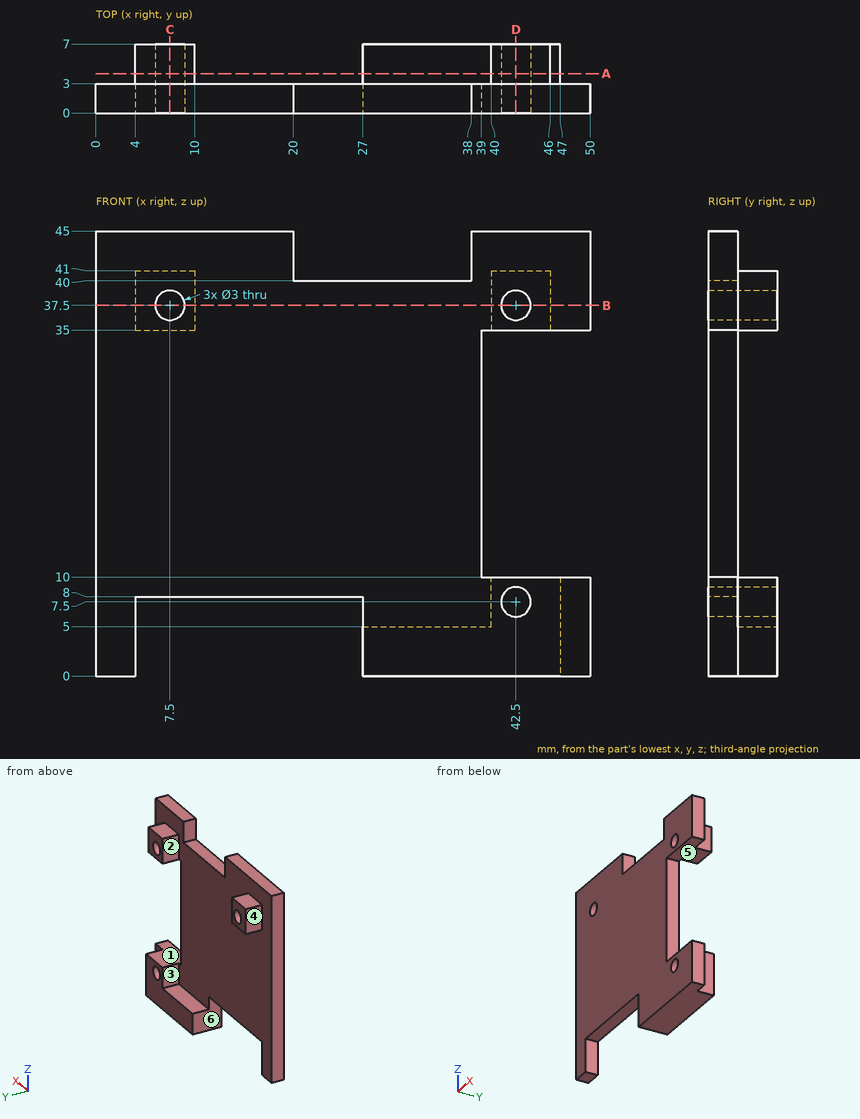
Part print with two shaded views. Sizes in mm from the minimum x, y, z corner. A direction names the side the tool comes from. Give positions to 0.01 mm unless a question says otherwise; leave off trailing zeros. Order: outer loops, then holes, each group sorted by start corner. A loop starts at its lowest first (then second) coordinate and runs counter-clockwise, first axis right, second up. Notation, with made-up numbers: M -40,-28.5 L 14,-28.5 A26 cw 14,7.5 Z; hole C 45,69.5 d5. An arc over 180 degrees is marked long. Write item = value, one per line.
Q1. Cut at C-C, the plane x = 7.5. List the corners of the cut face in (y, z), then the cut area to 3 significant figures.
Derived:
outline = M 0,8 L 3,8 L 3,35 L 7,35 L 7,36 L 0,36 Z; M 0,39 L 7,39 L 7,41 L 3,41 L 3,45 L 0,45 Z
area = 114 mm2
Q2. Cut at D-D, the plane x = 42.5. List the corners of the cut face in (y, z).
Derived:
outline = M 0,0 L 7,0 L 7,6 L 0,6 Z; M 0,9 L 7,9 L 7,10 L 0,10 Z; M 0,35 L 7,35 L 7,36 L 0,36 Z; M 0,39 L 7,39 L 7,41 L 3,41 L 3,45 L 0,45 Z
Q3. Drill centre lines: line 1 (X direction, y = 2.5, z = 37.5); line 2 (Z direction, x = 47.5, y = 1); line 3 (X direction, y = 2.5, z = 5.5). Where is each one in solid material? Low to high. Write a range as [from, to].
Derived:
line_1 = [0, 6], [9, 41], [44, 50]
line_2 = [0, 10], [35, 45]
line_3 = [0, 4], [27, 50]
Q4. Flat gauge pins, fed straight in: pin 1 (3.5 mm diameter, centred on x = 7.5, z = 37.5, fed in from +Y); pin 2 (1.2 mm diameter, centred on y = 5.5, z = 37, fed in from -X); pin 3 (3 mm diameter, centred on y = 5.5, z = 7, fed in from -X); pin 4 (1.2 mm diameter, centred on y = 5.5, z = 37, fed in from +X). Where does each tip first touch, or does it go through?
Derived:
pin_1 = 7
pin_2 = 4
pin_3 = 40
pin_4 = 46
Q5. Two-plate mould, pull along X, no slides. Class the marked faces 1, 2 and 3: pulls with the +X half, pulls with the -X half, needs draft (parallel to the pull), parting line crosses it, or undercut.
Derived:
face_1 = needs draft
face_2 = undercut
face_3 = pulls with the -X half
Q6. Tool access for the marked faces 4, 5 and 6: list every direction of +Z, -Z, +X, -X, +Y, -Y with a clear straight run to the whole face (end or side of a thin tool).
Derived:
face_4 = +Z, -Z, -X, +Y
face_5 = +X, +Y, -Y
face_6 = -Z, +Y, -Y
Q7. Cut at A-A, the plane y = 4. List the corners of the cut face in (x, z), then the cut area to 3 significant figures.
Derived:
outline = M 4,35 L 10,35 L 10,41 L 4,41 Z; M 27,0 L 47,0 L 47,10 L 40,10 L 40,5 L 27,5 Z; M 40,35 L 46,35 L 46,41 L 40,41 Z; hole C 7.5,37.5 d3; hole C 42.5,7.5 d3; hole C 42.5,37.5 d3
area = 186 mm2
Q8. Cut at B-B, the plane z = 37.5. List the corners of the cut face in (x, y), then the cut area to 3 significant figures.
Derived:
outline = M 0,0 L 6,0 L 6,7 L 4,7 L 4,3 L 0,3 Z; M 9,0 L 41,0 L 41,7 L 40,7 L 40,3 L 10,3 L 10,7 L 9,7 Z; M 44,0 L 50,0 L 50,3 L 46,3 L 46,7 L 44,7 Z
area = 156 mm2
